```python
from build123d import *

# Parameters (mm, degrees)
F1_DEPTH = 914.4
F3_DEPTH = 19.051
F5_DEPTH = 19.051


with BuildPart() as f1:
    # F0 (on Front) → F1 (new body)
    with BuildSketch(Plane.XZ):
        Polygon((0, 19.05), (0, 0), (19.05, 0), (19.05, 3.048), (3.048, 3.048), (3.048, 19.05), align=None)
    extrude(amount=F1_DEPTH)

    # F2 (on face) → F3 (cut, through all)
    with BuildSketch(Plane(origin=(0, 0, 0), x_dir=(1, 0, 0), z_dir=(0, 0, -1))):
        Polygon((19.05, 914.4), (0, 914.4), (19.05, 895.35), align=None)
    extrude(amount=-F3_DEPTH, mode=Mode.SUBTRACT)

    # F4 (on face) → F5 (cut, through all)
    with BuildSketch(Plane(origin=(0, 0, 0), x_dir=(1, 0, 0), z_dir=(0, 0, -1))):
        Polygon((19.05, 19.05), (0, 0), (19.05, 0), align=None)
    extrude(amount=-F5_DEPTH, mode=Mode.SUBTRACT)


solid = f1.part
```
Geometry: final body of the model. Coordinates: model frame, mm. A direction names the side the tool comes from. Round coordinates to 2 decimals unless told otherwise and drop trailing zeros. Write each loop counter-clockwise with the first axis right and the second up, starting at its lowest first coordinate (ties: lowest second). Pieces come first, ordered by that corner, then holes. Notation, with made-up numbers: M -9,-16.5 L 41,-16.5 A10 cw 41,-1.5 Z; hole C 35.5,63 d10. An arc over 180 degrees is marked long. Answer in a Markdown table with one row per item. Add a question column.
(1) Cut plane C-C, the plane x = 13.25. Return the cut outline in (y, z).
(2) Reachability of faces 4 (the face through (11, -451, 3.048)), 5 (the face through (9, -451, 0)) from +Z, -Z, +X, -X, +Y, -Y: full face, straight path, thin tool, end or side. Return the list, or none.
(3) Draft query along Y for faces 1 (the face through (3.048, -451, 11)), 2 (the face through (5.2, -909.2, 0.9)), 3 (the face through (5, -5, 2)). Return one class per face: pulls with the +Y half, pulls with the -Y half, needs draft (parallel to the pull), parting line crosses it, or undercut.
(4) Cut plane A-A, the plane y = -389.5. Return the cut outline in (x, z), then the cut area to 3 significant figures.
(5) Ray query, L1, parallel to X at y = -830, z = 6.25; L2, parallel to Y at x = 4.25, z = 1.25. Return the intervals inside material, ascending.
(6) Contact query for a flat-ended pin moving along its axis: pin 1 (5 mm diameter, centred on x = 17, y = -450.5, fed in from +Z). Output: stop coordinate, or through.
(7) Cut plane B-B, the plane z = 8.5. Return the cut outline in (x, y).
Established:
| question | item | result |
|---|---|---|
| 1 | outline | M -901.15,0 L -13.25,0 L -13.25,3.05 L -901.15,3.05 Z |
| 2 | face 4 | +Z, +X, +Y, -Y |
| 2 | face 5 | -Z, +X, -X, +Y, -Y |
| 3 | face 1 | needs draft |
| 3 | face 2 | pulls with the -Y half |
| 3 | face 3 | pulls with the +Y half |
| 4 | outline | M 0,0 L 19.05,0 L 19.05,3.05 L 3.05,3.05 L 3.05,19.05 L 0,19.05 Z |
| 4 | area | 107 mm² |
| 5 | L1 | 0 to 3.05 |
| 5 | L2 | -910.15 to -4.25 |
| 6 | pin 1 | z = 3.05 |
| 7 | outline | M 0,-914.4 L 3.05,-911.35 L 3.05,-3.05 L 0,0 Z |
